```python
from build123d import *

# Parameters (mm, degrees)
ESQUISSE1_R             = 47.5
BOSS_EXTRU_1_DEPTH      = 10
ESQUISSE3_W             = 100
ESQUISSE3_H             = 10
ENL_V_MAT_EXTRU_1_DEPTH = 11
ESQUISSE4_R             = 2.5
ENL_V_MAT_EXTRU_2_DEPTH = 11
ESQUISSE6_W             = 75
ESQUISSE6_H             = 120
BOSS_EXTRU_2_DEPTH      = 10
ESQUISSE7_W             = 10
ESQUISSE7_H             = 50
ESQUISSE7_W_2           = 30
ESQUISSE7_H_2           = 9.570800355
ENL_V_MAT_EXTRU_3_DEPTH = 10
ENL_V_MAT_EXTRU_6_DEPTH = 10
ESQUISSE12_W            = 10
ESQUISSE12_H            = 30
ENL_V_MAT_EXTRU_7_DEPTH = 10


with BuildPart() as part:
    # Esquisse1 → Boss.-Extru.1 (new body)
    with BuildSketch(Plane.XY):
        Polygon((-310, -75.642859016), (0, 414.561180135), (310, -75.642859016), align=None)
        with Locations((-157.5, 0)):
            Circle(ESQUISSE1_R, mode=Mode.SUBTRACT)
        with Locations((-52.5, 0)):
            Circle(ESQUISSE1_R, mode=Mode.SUBTRACT)
        with Locations((52.5, 0)):
            Circle(ESQUISSE1_R, mode=Mode.SUBTRACT)
        with Locations((157.5, 0)):
            Circle(ESQUISSE1_R, mode=Mode.SUBTRACT)
        with Locations((-105, 90.932667397)):
            Circle(ESQUISSE1_R, mode=Mode.SUBTRACT)
        with Locations((0, 90.932667397)):
            Circle(ESQUISSE1_R, mode=Mode.SUBTRACT)
        with Locations((105, 90.932667397)):
            Circle(ESQUISSE1_R, mode=Mode.SUBTRACT)
        with Locations((-52.5, 181.865334795)):
            Circle(ESQUISSE1_R, mode=Mode.SUBTRACT)
        with Locations((52.5, 181.865334795)):
            Circle(ESQUISSE1_R, mode=Mode.SUBTRACT)
        with Locations((0, 272.798002192)):
            Circle(ESQUISSE1_R, mode=Mode.SUBTRACT)
    extrude(amount=BOSS_EXTRU_1_DEPTH)

    # Esquisse3 → Enlèv. mat.-Extru.1 (cut, through all)
    with BuildSketch(Plane.XY.offset(10)):
        Polygon((-269.913793103, -12.254405678), (-261.461999325, -17.599233264), (-208.013723463, 66.918704521), (-216.465517241, 72.263532107), align=None)
        Polygon((-181.724137931, 127.200191667), (-173.272344153, 121.855364081), (-119.82406829, 206.373301865), (-128.275862069, 211.718129452), align=None)
        Polygon((-93.534482759, 266.654789012), (-85.08268898, 261.309961425), (-31.634413118, 345.82789921), (-40.086206897, 351.172726796), align=None)
        Polygon((269.913793103, -12.254405678), (261.461999325, -17.599233264), (208.013723463, 66.918704521), (216.465517241, 72.263532107), align=None)
        Polygon((181.724137931, 127.200191667), (173.272344153, 121.855364081), (119.82406829, 206.373301865), (128.275862069, 211.718129452), align=None)
        Polygon((93.534482759, 266.654789012), (85.08268898, 261.309961425), (31.634413118, 345.82789921), (40.086206897, 351.172726796), align=None)
        with Locations((-160, -70.642859016)):
            Rectangle(ESQUISSE3_W, ESQUISSE3_H)
        with Locations((160, -70.642859016)):
            Rectangle(ESQUISSE3_W, ESQUISSE3_H)
    extrude(amount=-ENL_V_MAT_EXTRU_1_DEPTH, mode=Mode.SUBTRACT)

    # Esquisse4 → Enlèv. mat.-Extru.2 (cut, through all)
    with BuildSketch(Plane.XY.offset(10)):
        with Locations((-157.5, -55.642859016)):
            Circle(ESQUISSE4_R)
        with Locations((-52.5, -55.642859016)):
            Circle(ESQUISSE4_R)
        with Locations((52.5, -55.642859016)):
            Circle(ESQUISSE4_R)
        with Locations((157.5, -55.642859016)):
            Circle(ESQUISSE4_R)
        with Locations((-105, 29.047375097)):
            Circle(ESQUISSE4_R)
        with Locations((0, 29.047375097)):
            Circle(ESQUISSE4_R)
        with Locations((105, 29.047375097)):
            Circle(ESQUISSE4_R)
        with Locations((-52.5, 119.980042494)):
            Circle(ESQUISSE4_R)
        with Locations((52.5, 119.980042494)):
            Circle(ESQUISSE4_R)
        with Locations((0, 210.912709891)):
            Circle(ESQUISSE4_R)
    extrude(amount=-ENL_V_MAT_EXTRU_2_DEPTH, mode=Mode.SUBTRACT)

    # Esquisse6 → Boss.-Extru.2 (add)
    with BuildSketch(Plane.XY.offset(10)):
        with Locations((0, -135.642859016)):
            Rectangle(ESQUISSE6_W, ESQUISSE6_H)
    extrude(amount=-BOSS_EXTRU_2_DEPTH)

    # Esquisse7 → Enlèv. mat.-Extru.3 (cut)
    with BuildSketch(Plane.XY.offset(10)):
        with Locations((-32.5, -135.642859016)):
            Rectangle(ESQUISSE7_W, ESQUISSE7_H)
        with Locations((1.495284743, -190.857458839)):
            Rectangle(ESQUISSE7_W_2, ESQUISSE7_H_2)
        with Locations((32.5, -135.642859016)):
            Rectangle(ESQUISSE7_W, ESQUISSE7_H)
    extrude(amount=-ENL_V_MAT_EXTRU_3_DEPTH, mode=Mode.SUBTRACT)

    # Esquisse11 → Enlèv. mat.-Extru.6 (cut)
    with BuildSketch(Plane.XY.offset(10)):
        Polygon((0, 414.561180135), (0, 109.461180135), (-346.154388362, 109.461180135), (-346.154388362, -222.549126753), (369.346533709, -222.549126753), (369.346533709, 414.561180135), align=None)
    extrude(amount=-ENL_V_MAT_EXTRU_6_DEPTH, mode=Mode.SUBTRACT)

    # Esquisse12 → Enlèv. mat.-Extru.7 (cut)
    with BuildSketch(Plane.XY.offset(10)):
        with Locations((-5, 359.561180135)):
            Rectangle(ESQUISSE12_W, ESQUISSE12_H)
    extrude(amount=-ENL_V_MAT_EXTRU_7_DEPTH, mode=Mode.SUBTRACT)


solid = part.part
```
Could you check a few things on this model? Use its own coordinates, in mm. A direction names the side the tool comes from. Coordinates: 2 decimals unless noted, no trailing zeros. Write each loop counter-clockwise with the first axis right and the second up, starting at its lowest first coordinate (ties: lowest second). Pieces come first, ordered by that corner, then holes. Notation, with made-up numbers: (63, -19) -> (88, -19) arc R24 ccw to (88, 7) -> close; hole circle Ø8 at (60.5, -37). An arc over 180 degrees is marked (long way). Return JSON: item names as keys, results as strings.
(1) Imagine slicing it at A-A, the plane y = 170. Please give me the cut outline in (x, z), then the cut area to 3 significant figures.
Numbers:
{"outline": "(-142.83, 0) -> (-98.49, 0) -> (-98.49, 10) -> (-142.83, 10) -> close; (-6.51, 0) -> (0, 0) -> (0, 10) -> (-6.51, 10) -> close", "area": "508 mm2"}
(2) Imagine slicing it at C-C, the plane x = -108.5. Please give me the cut outline in (y, z).
Numbers:
{"outline": "(138.3, 0) -> (242.99, 0) -> (242.99, 10) -> (138.3, 10) -> close"}
(3) We'd pull the mould along X, two halves only. Please class faces 4 (the flat face through (-5, 344.561, 5)), 5 (the cylindrical face through (-58.68, 228.96, 4.93)), 6 (the flat face through (-10, 359, 5)): +X half, -X half, draft (parallel to the pull), parting line (faces both ways), or undercut.
Numbers:
{"face 4": "draft", "face 5": "undercut", "face 6": "+X half"}
(4) Imagine slicing it at B-B, the plane z = 3.5. Please give me the cut outline in (x, y), then the cut area to 3 significant figures.
Numbers:
{"outline": "(-192.94, 109.46) -> (-148.74, 109.46) arc R47.5 cw to (-61.26, 109.46) -> (-43.74, 109.46) arc R47.5 cw to (0, 138.43) -> (0, 208.41) arc R2.5 cw to (0, 213.41) -> (0, 225.3) arc R47.5 cw to (0, 320.3) -> (0, 344.56) -> (-10, 344.56) -> (-10, 374.56) -> (0, 374.56) -> (0, 414.56) -> (-40.09, 351.17) -> (-31.63, 345.83) -> (-85.08, 261.31) -> (-93.53, 266.65) -> (-128.28, 211.72) -> (-119.82, 206.37) -> (-173.27, 121.86) -> (-181.72, 127.2) -> close; hole circle Ø95 at (-52.5, 181.87); hole circle Ø5 at (-52.5, 119.98)", "area": "13,700 mm2"}
(5) Imagine slicing it at D-D, the plane y = 300. Please give me the cut outline in (x, z), then the cut area to 3 significant figures.
Numbers:
{"outline": "(-60.62, 0) -> (-38.94, 0) -> (-38.94, 10) -> (-60.62, 10) -> close", "area": "217 mm2"}
(6) I need wall thicknesses on L1, parallel to Y at x = -11, z = 8.5; L2, parallel to Y at x = -12, z = 6; L3, parallel to Y at x = -121, z = 6. Which ranges of each line are inside material? Lowest first, please.
Numbers:
{"L1": "y = 137.14 to 158.76, 204.97 to 226.59, 319.01 to 397.17", "L2": "y = 136.89 to 157.05, 206.68 to 226.84, 318.76 to 395.59", "L3": "y = 135.66 to 204.51, 207.12 to 223.22"}
(7) I'm going to push flat-ended pins straight in: pin 1 (2 mm diameter, centred on x = -70.5, z = 3, fed in from +Y); pin 2 (5 mm diameter, centred on x = -4.5, z = 3.5, fed in from -Y); pin 3 (2 mm diameter, centred on x = -84.5, z = 7, fed in from +Y). Where does each tip first touch, or does it pass through?
Numbers:
{"pin 1": "stops at y = 285.95", "pin 2": "stops at y = 137.91", "pin 3": "stops at y = 263.81"}
(8) Which directions (+Z, -Z, +X, -X, +Y, -Y) give clear straight access to the entire face, cutting with the end or side of a thin tool? Please do faces 1 (the flat face through (-89.37, 264.02, 5.07)), 2 (the flat face through (0, 333, 5)), 3 (the flat face through (-123.99, 209.01, 5.07)).
Numbers:
{"face 1": "+Z, -Z, +Y", "face 2": "+Z, -Z, +X, +Y, -Y", "face 3": "+Z, -Z, -X"}
